Build history of the part. All positions in model axes, mm. A direction names the side the tool comes from. Give positions to 0.01 mm unless a question says otherwise; leave off trailing zeros. Order: outer loops, then holes, each group sorted by start corner. A loop starts at its lowest first (then second) coordinate and runs counter-clockwise, first axis right, second up. Notation, with made-up numbers: (-9.5, -0.5) - (41.5, -0.5) arc R10 cw to (41.5, 3.5) - close; hole circle Ø10 at (-3, 49.25). An arc over 180 degrees is marked (long way). Write each question's results on one line, items separated by ' | '. Start each with the question number.
from build123d import *

# Parameters (mm, degrees)
SKETCH_1_R      = 1
SKETCH_1_R_2    = 1.5
SKETCH_1_W      = 1.2
SKETCH_1_H      = 34.088931988
EXTRUDE_1_DEPTH = 2


with BuildPart() as part:
    # 草图1 → 凸台-拉伸1 (new body)
    with BuildSketch(Plane.XY):
        with BuildLine():
            Line((-12.91723747, 0), (12.91723747, 0))
            ThreePointArc((12.91723747, 0), (17.453878353, 2.073310619), (18.855230664, 6.860370167))
            Line((18.855230664, 6.860370167), (9.744693373, 69.738315612))
            ThreePointArc((9.744693373, 69.738315612), (7.73338956, 73.414586328), (3.806700178, 74.877945445))
            Line((3.806700178, 74.877945445), (0, 74.877945445))
            Line((0, 74.877945445), (-3.806700178, 74.877945445))
            ThreePointArc((-3.806700178, 74.877945445), (-7.73338956, 73.414586328), (-9.744693373, 69.738315612))
            Line((-9.744693373, 69.738315612), (-18.855230664, 6.860370167))
            ThreePointArc((-18.855230664, 6.860370167), (-17.453878353, 2.073310619), (-12.91723747, 0))
        make_face()
        with Locations((11.7, 4)):
            Circle(SKETCH_1_R, mode=Mode.SUBTRACT)
        with Locations((-11.7, 4)):
            Circle(SKETCH_1_R, mode=Mode.SUBTRACT)
        with Locations((-3, 10)):
            Circle(SKETCH_1_R_2, mode=Mode.SUBTRACT)
        with Locations((3, 10)):
            Circle(SKETCH_1_R_2, mode=Mode.SUBTRACT)
        with Locations((-6.2, 53.192179666)):
            Rectangle(SKETCH_1_W, SKETCH_1_H, mode=Mode.SUBTRACT)
    extrude(amount=EXTRUDE_1_DEPTH)


solid = part.part
Item 1: Cut at C-C, the plane y = 51.5. List the corners of the cut face in (x, z), then the cut area to 3 significant figures.
Item 2: Cut at A-A, the plane z = 0.4. List the corners of the cut face in (x, y), then the cut area to 3 significant figures.
Item 3: Two-plate mould, pull along Y, no slides. Class faces 3 (the cylindrical face through (7.779, 73.375, 0.986)), 4 (the flat face through (0, 38, 0)), 5 (the flat face through (-5.6, 53, 1)): +Y half, -Y half, draft (parallel to the pull), parting line (faces both ways), or undercut.
Item 4: Probe line 1 along Y through (x, z) = (3, 1.25); line 2 along X through (y, z) = (40, 0.5); line 3 along Y through (x, z) = (-2.5, 1.55). List the from-to ranges inside material, lowest first. Write a range as from..to.
Item 5: Cut at D-D, the plane y = 10. List the corners of the cut face in (x, z), then the cut area to 3 significant figures.
Item 6: Which spindle directions (+Z, -Z, +X, -X, +Y, -Y) get a long thin tool onto all of the face, cutting with end or side? Do faces 1 (the flat face through (-6.8, 53, 1)), 2 (the cylindrical face through (-7.69, 73.45, 0.99)). Say none if no direction does.
Item 7: Flat gauge pins, fed straight in: pin 1 Ø2.5 at (x, y) = (3, 10) entering from -Z; pin 2 Ø1 at (y, z) = (47.5, 1.5) entering from -X. Where does each tip first touch, or does it go through?
Item 8: Cut at B-B, the plane x = 3. List the corners of the cut face in (y, z), then the cut area to 3 significant figures.
Values found:
1) outline: (-12.39, 0) - (-6.8, 0) - (-6.8, 2) - (-12.39, 2) - close; (-5.6, 0) - (12.39, 0) - (12.39, 2) - (-5.6, 2) - close | area: 47.1 mm2
2) outline: (-18.86, 6.86) arc R6 ccw to (-12.92, 0) - (12.92, 0) arc R6 ccw to (18.86, 6.86) - (9.74, 69.74) arc R6 ccw to (3.81, 74.88) - (-3.81, 74.88) arc R6 ccw to (-9.74, 69.74) - close; hole circle Ø2 at (-11.7, 4); hole (-6.8, 36.15) - (-5.6, 36.15) - (-5.6, 70.24) - (-6.8, 70.24) - close; hole circle Ø3 at (-3, 10); hole circle Ø3 at (3, 10); hole circle Ø2 at (11.7, 4) | area: 2,070 mm2
3) face 3: +Y half | face 4: draft | face 5: undercut
4) line 1: y = 0..8.5, 11.5..74.88 | line 2: x = -14.05..-6.8, -5.6..14.05 | line 3: y = 0..8.59, 11.41..74.88
5) outline: (-18.4, 0) - (-4.5, 0) - (-4.5, 2) - (-18.4, 2) - close; (-1.5, 0) - (1.5, 0) - (1.5, 2) - (-1.5, 2) - close; (4.5, 0) - (18.4, 0) - (18.4, 2) - (4.5, 2) - close | area: 61.6 mm2
6) face 1: +Z, -Z | face 2: +Z, -Z, -X, +Y
7) pin 1: passes through | pin 2: stops at x = -13.04
8) outline: (0, 0) - (8.5, 0) - (8.5, 2) - (0, 2) - close; (11.5, 0) - (74.88, 0) - (74.88, 2) - (11.5, 2) - close | area: 144 mm2
